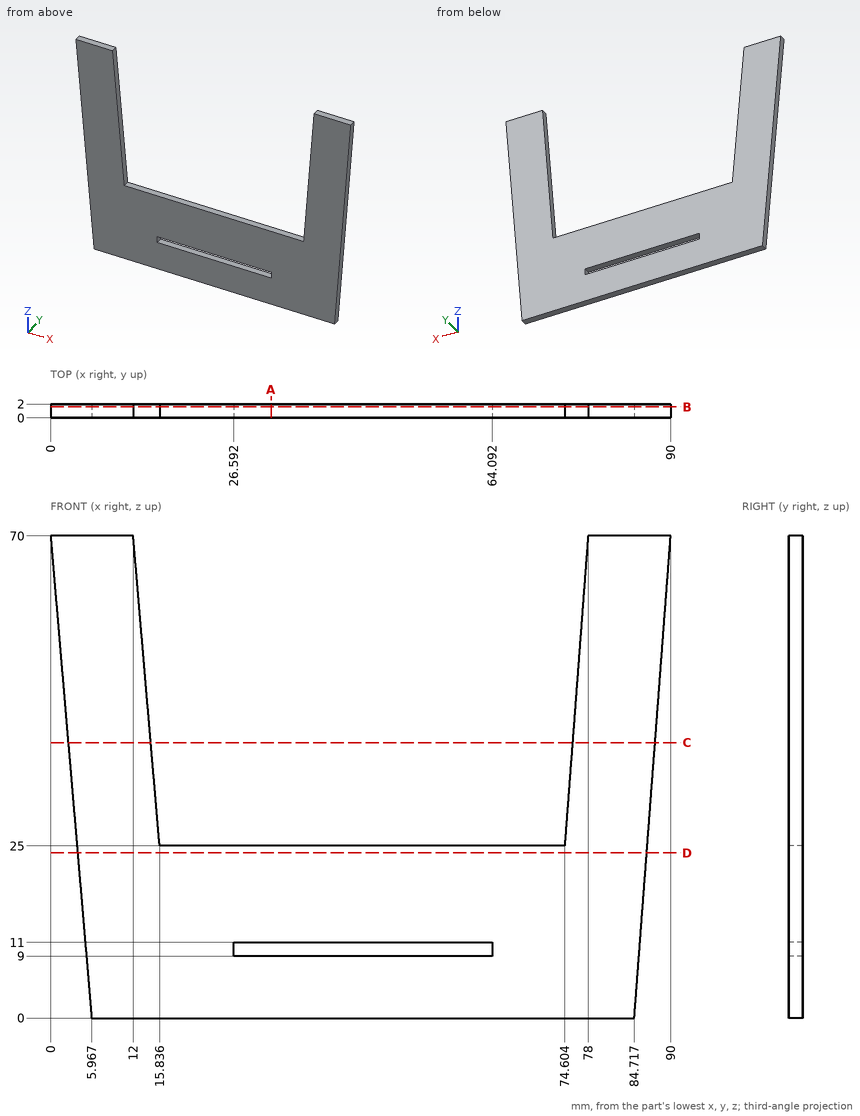
Can you work these out from the drawing? Everything is in mm from the part's minimum corner. Round coordinates to 2 decimals unless told otherwise and drop trailing zeros. Write each loop counter-clockwise with the first axis right and the second up, starting at its lowest first coordinate (ties: lowest second). Pieces come first, ordered by that corner, then holes. Notation, with made-up numbers: (5.5, 84.25) - (21.5, 84.25) arc R15 ccw to (21.5, 113.25) - close; hole circle Ø4 at (48, 46). An arc over 180 degrees is marked (long way). Use a Markdown table: item, result.
Q1. I want a section at B-B (y = 1.6). List the corners of the cut face in (x, z) for me.
Output values:
| item | result |
|---|---|
| outline | (0, 70) - (5.97, 0) - (84.72, 0) - (90, 70) - (78, 70) - (74.6, 25) - (15.84, 25) - (12, 70) - close; hole (26.59, 9) - (64.09, 9) - (64.09, 11) - (26.59, 11) - close |
Q2. I want a section at C-C (z = 40). List the corners of the cut face in (x, y) for me, plus the area to 3 significant figures.
Output values:
| item | result |
|---|---|
| outline | (2.56, 0) - (14.56, 0) - (14.56, 2) - (2.56, 2) - close; (75.74, 0) - (87.74, 0) - (87.74, 2) - (75.74, 2) - close |
| area | 48.0 mm2 |
Q3. I want a section at A-A (x = 32). List the corners of the cut face in (y, z) for me, plus the area to 3 significant figures.
Output values:
| item | result |
|---|---|
| outline | (0, 0) - (2, 0) - (2, 9) - (0, 9) - close; (0, 11) - (2, 11) - (2, 25) - (0, 25) - close |
| area | 46.0 mm2 |
Q4. Please list where these lines run through material, in increasing order: L1, parallel to Z at x = 31, y = 1.2; L2, parallel to X at y = 1.15, z = 41; L3, parallel to Z at x = 74, y = 1.25.
Output values:
| item | result |
|---|---|
| L1 | 0 to 9, 11 to 25 |
| L2 | 2.47 to 14.47, 75.81 to 87.81 |
| L3 | 0 to 25 |
Q5. For pin 1 (0.6 mm diameter, centred on y = 1.5, z = 9.5, fed in from +X), with a flat end and sliding along its axis, tell me the tip position at first contact or that it passes through.
Output values:
| item | result |
|---|---|
| pin 1 | x = 85.46 |
Q6. I want a section at D-D (z = 24). List the corners of the cut face in (x, y) for me.
Output values:
| item | result |
|---|---|
| outline | (3.92, 0) - (86.53, 0) - (86.53, 2) - (3.92, 2) - close |
